from build123d import *

# Parameters (mm, degrees)
F1_DEPTH  = 3.175
F2_W      = 194
F2_H      = 113
F3_DEPTH  = 15.875
F5_DEPTH  = 12.7
F7_DEPTH  = 3.175
F9_DEPTH  = 3.175
F10_DEPTH = 6.35


with BuildPart() as f1:
    # F0 (on Front) → F1 (new body)
    with BuildSketch(Plane.XZ):
        with BuildLine():
            ThreePointArc((79.375, 48.41875), (77.5151280605, 52.9088780605), (73.025, 54.76875))
            Line((73.025, 54.76875), (-73.025, 54.76875))
            ThreePointArc((-73.025, 54.76875), (-77.5151280605, 52.9088780605), (-79.375, 48.41875))
            Line((-79.375, 48.41875), (-79.375, -48.41875))
            ThreePointArc((-79.375, -48.41875), (-77.5151280605, -52.9088780605), (-73.025, -54.76875))
            Line((-73.025, -54.76875), (73.025, -54.76875))
            ThreePointArc((73.025, -54.76875), (77.5151280605, -52.9088780605), (79.375, -48.41875))
            Line((79.375, -48.41875), (79.375, 48.41875))
        make_face()
    extrude(amount=F1_DEPTH)

    # F2 (on face) → F3 (join)
    with BuildSketch(Plane.XZ.offset(3.175)):
        Rectangle(F2_W, F2_H)
    extrude(amount=F3_DEPTH)

    # F4 (on face) → F5 (cut)
    with BuildSketch(Plane.XZ.offset(19.05)):
        with BuildLine():
            Line((67.95, 46.5), (-67.95, 46.5))
            ThreePointArc((-67.95, 46.5), (-81.4203841816, 40.9203841816), (-87, 27.45))
            Line((-87, 27.45), (-87, -27.45))
            ThreePointArc((-87, -27.45), (-81.4203841816, -40.9203841816), (-67.95, -46.5))
            Line((-67.95, -46.5), (67.95, -46.5))
            ThreePointArc((67.95, -46.5), (81.4203841816, -40.9203841816), (87, -27.45))
            Line((87, -27.45), (87, 27.45))
            ThreePointArc((87, 27.45), (81.4203841816, 40.9203841816), (67.95, 46.5))
        make_face()
    extrude(amount=-F5_DEPTH, mode=Mode.SUBTRACT)

    # F6 (on face) → F7 (join)
    with BuildSketch(Plane.XZ.offset(6.35)):
        with BuildLine():
            Line((66.2125, 41.5), (-66.2125, 41.5))
            ThreePointArc((-66.2125, 41.5), (-76.3152881362, 37.3152881362), (-80.5, 27.2125))
            Line((-80.5, 27.2125), (-80.5, -27.2125))
            ThreePointArc((-80.5, -27.2125), (-76.3152881362, -37.3152881362), (-66.2125, -41.5))
            Line((-66.2125, -41.5), (66.2125, -41.5))
            ThreePointArc((66.2125, -41.5), (76.3152881362, -37.3152881362), (80.5, -27.2125))
            Line((80.5, -27.2125), (80.5, 27.2125))
            ThreePointArc((80.5, 27.2125), (76.3152881362, 37.3152881362), (66.2125, 41.5))
        make_face()
    extrude(amount=F7_DEPTH)

    # F8 (on face) → F9 (cut)
    with BuildSketch(Plane.XZ.offset(9.525)):
        with BuildLine():
            Line((65.88125, 34.13125), (-65.88125, 34.13125))
            ThreePointArc((-65.88125, 34.13125), (-71.4939100757, 31.8064100757), (-73.81875, 26.19375))
            Line((-73.81875, 26.19375), (-73.81875, -26.19375))
            ThreePointArc((-73.81875, -26.19375), (-71.4939100757, -31.8064100757), (-65.88125, -34.13125))
            Line((-65.88125, -34.13125), (65.88125, -34.13125))
            ThreePointArc((65.88125, -34.13125), (71.4939100757, -31.8064100757), (73.81875, -26.19375))
            Line((73.81875, -26.19375), (73.81875, 26.19375))
            ThreePointArc((73.81875, 26.19375), (71.4939100757, 31.8064100757), (65.88125, 34.13125))
        make_face()
    extrude(amount=-F9_DEPTH, mode=Mode.SUBTRACT)

    # F10 (add): a face of the model
    f10_faces = [f1.faces().sort_by_distance(p)[0] for p in [
        (85.0270580343, -6.35, 0),
    ]]
    extrude(f10_faces, amount=F10_DEPTH)


solid = f1.part
Work out the finished part from the listing and answer in its coordinate system (mm). A direction names the side the tool comes from. Round coordinates to 2 decimals unless told otherwise and drop trailing zeros. Write each loop counter-clockwise with the first axis right and the second up, starting at its lowest first coordinate (ties: lowest second). Pieces come first, ordered by that corner, then holes. Notation, with made-up numbers: M 6,3 L 23,3 A17 cw 23,19 Z; hole C 45,36.5 d6. An arc over 180 degrees is marked long. Use a Markdown table: item, result.
1) Flat-ended cylindrical pins translate along their axes: pin 1 (3.5 mm diameter, centred on y = -1.5, z = -9.5, fed in from -X); pin 2 (1 mm diameter, centred on x = -31, y = -1, fed in from -Z); pin 3 (10 mm diameter, centred on x = -25, z = -21.5, fed in from -Y). Find the tip coordinate at first contact, or state that the pin passes through.
Taken from the geometry:
| item | result |
|---|---|
| pin 1 | stops at x = -97 |
| pin 2 | stops at z = -54.77 |
| pin 3 | stops at y = -6.35 |
2) The part is cut by section C-C on x = 76. Give the vertices of the cut face in (y, z) (3 decimals), plus the area to 3 significant figures.
Taken from the geometry:
| item | result |
|---|---|
| outline | M -19.05,-56.5 L -3.175,-56.5 L -3.175,-54.029 L 0,-54.029 L 0,54.029 L -3.175,54.029 L -3.175,56.5 L -19.05,56.5 L -19.05,44.716 L -12.7,44.716 L -12.7,37.621 L -9.525,37.621 L -9.525,-37.621 L -12.7,-37.621 L -12.7,-44.716 L -19.05,-44.716 Z |
| area | 1,330 mm2 |
3) Consider line 1 (X direction, y = -18.5, z = -24); line 2 (X direction, y = -10.5, z = -16); line 3 (Z direction, x = -48, y = -10.25). Determine where each line is inside the solid, lowest interval first. Write a range as [from, to].
Taken from the geometry:
| item | result |
|---|---|
| line 1 | x = [-97, -87], [87, 97] |
| line 2 | x = [-97, -80.5], [80.5, 97] |
| line 3 | z = [-56.5, -41.5], [41.5, 56.5] |
4) The part is cut by section B-B on z = 3.5. Give the vertices of the cut face in (x, y) (3 decimals), plus the area to 3 significant figures.
Taken from the geometry:
| item | result |
|---|---|
| outline | M -97,-19.05 L -87,-19.05 L -87,-12.7 L -80.5,-12.7 L -80.5,-9.525 L -73.819,-9.525 L -73.819,-6.35 L 73.819,-6.35 L 73.819,-9.525 L 80.5,-9.525 L 80.5,-12.7 L 87,-12.7 L 87,-19.05 L 97,-19.05 L 97,-3.175 L 79.375,-3.175 L 79.375,0 L -79.375,0 L -79.375,-3.175 L -97,-3.175 Z |
| area | 1,500 mm2 |
5) The part is cut by section D-D on z = -39.5. Give the vertices of the cut face in (x, y) (3 decimals).
Taken from the geometry:
| item | result |
|---|---|
| outline | M -97,-19.05 L -82.705,-19.05 L -82.705,-12.7 L -73.503,-12.7 L -73.503,-9.525 L 73.503,-9.525 L 73.503,-12.7 L 82.705,-12.7 L 82.705,-19.05 L 97,-19.05 L 97,-3.175 L 79.375,-3.175 L 79.375,0 L -79.375,0 L -79.375,-3.175 L -97,-3.175 Z |
6) The part is cut by section A-A on x = -54. Give the vertices of the cut face in (y, z) (3 decimals).
Taken from the geometry:
| item | result |
|---|---|
| outline | M -19.05,-56.5 L -3.175,-56.5 L -3.175,-54.769 L 0,-54.769 L 0,54.769 L -3.175,54.769 L -3.175,56.5 L -19.05,56.5 L -19.05,46.5 L -12.7,46.5 L -12.7,41.5 L -9.525,41.5 L -9.525,34.131 L -6.35,34.131 L -6.35,-34.131 L -9.525,-34.131 L -9.525,-41.5 L -12.7,-41.5 L -12.7,-46.5 L -19.05,-46.5 Z |
7) Which of the six approach directions +Z, -Z, +X, -X, +Y, -Y give full straight-line access (tool end or side, diameter ignored) to faces 1 (the face through (76.2, -11.09, -37.43)), 2 (the face through (-77.564, -1.565, -52.859)), 3 (the face through (0, -19.05, -50))?
Taken from the geometry:
| item | result |
|---|---|
| face 1 | -Y |
| face 2 | -Z, -X, +Y |
| face 3 | +Z, -Z, +X, -X, -Y |
